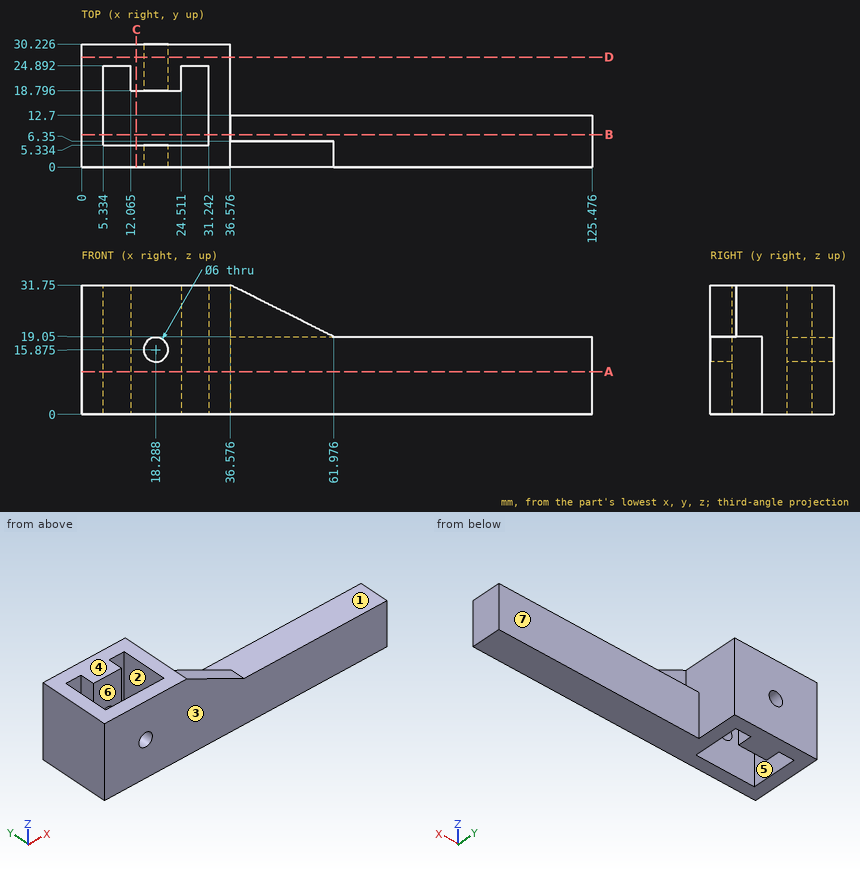
Answer from the drawing. Dimensions are ordinates in mm from the lowest x, y and z of the part. A direction names the side the tool comes from. Give positions to 0.01 mm unless a question says otherwise; leave off trailing zeros. Write each loop counter-clockwise with the first axis right and the second up, starting at its lowest first coordinate (ties: lowest second). Pieces come first, ordered by that corner, then holes. Notation, with made-up numbers: M 22,75.25 L 34,75.25 A27 cw 34,106.25 Z; hole C 58.25,67.5 d7. An arc over 180 degrees is marked long. Answer as CSV lines item,"result".
Q1. A tool of negligible diameter and unlimited length cuts with its end or side. For the marked faces 1, 2 and 3, from which of +Z, -Z, +X, -X, +Y, -Y can it reach the whole face along a straight path? Write none if from no direction.
A:
face 1,"+Z, +X, +Y"
face 2,"+Z, -Z"
face 3,"+Z, -Z, +X, -X, -Y"
Q2. A cutting plane is placed at A-A on z = 10.5. Write down the section's boundary in (x, y) (3 decimals), plus the area to 3 significant figures.
A:
outline,"M 0,0 L 125.476,0 L 125.476,12.7 L 36.576,12.7 L 36.576,30.226 L 0,30.226 Z; hole M 5.334,5.334 L 31.242,5.334 L 31.242,24.892 L 24.511,24.892 L 24.511,18.796 L 12.065,18.796 L 12.065,24.892 L 5.334,24.892 Z"
area,"1,800 mm²"
Q3. Given P1, Ø1, axis at y = 18, z = 13, coming from the +X side; P2, Ø14, axis at x = 80.5, y = 7.5, coming from the +Z side; P3, Ø14, axis at x = 44.5, z = 26, coming from the +Y side, each flat-ended and moving along its own axis, determine where each tip first touches the part or whether it passes through.
A:
P1,"stops at x = 36.58"
P2,"stops at z = 19.05"
P3,"stops at y = 12.7"
Q4. Find the intervals of material crossed by probe 1 along X at (y, z) = (8, 19); probe 2 along Y at (x, z) = (28.5, 7); probe 3 along X at (y, z) = (17, 12), in increasing order. Write a range as [from, to].
A:
probe 1,"x = [0, 5.33], [31.24, 125.48]"
probe 2,"y = [0, 5.33], [24.89, 30.23]"
probe 3,"x = [0, 5.33], [31.24, 36.58]"
Q5. The mould has two halves that part along Y. Classify the marked faces 4, 5, 6 and 7: +Y half, -Y half, draft (parallel to the pull), parting line (faces both ways), or undercut.
A:
face 4,"draft"
face 5,"undercut"
face 6,"undercut"
face 7,"+Y half"
Q6. A cutting plane is placed at D-D on y = 27. Write down the section's boundary in (x, z) (3 decimals), plus the area to 3 significant figures.
A:
outline,"M 0,0 L 36.576,0 L 36.576,31.75 L 0,31.75 Z; hole C 18.288,15.875 d6"
area,"1,130 mm²"
Q7. A cutting plane is placed at C-C on x = 13.5. Write down the section's boundary in (y, z), plus the area to 3 significant figures.
A:
outline,"M 0,0 L 5.33,0 L 5.33,31.75 L 0,31.75 Z; M 18.8,0 L 30.23,0 L 30.23,31.75 L 18.8,31.75 Z"
area,"532 mm²"
Q8. A cutting plane is placed at B-B on y = 8. Write down the section's boundary in (x, z), plus the area to 3 significant figures.
A:
outline,"M 0,0 L 5.33,0 L 5.33,31.75 L 0,31.75 Z; M 31.24,0 L 125.48,0 L 125.48,19.05 L 36.58,19.05 L 36.58,31.75 L 31.24,31.75 Z"
area,"2,030 mm²"
